Here's how the part is built. I have some questions about the finished solid (model axes, mm). A direction names the side the tool comes from. Give positions to 0.01 mm unless a question says otherwise; leave off trailing zeros. Loops run counter-clockwise (first coordinate to the right, second up) from the corner with the lowest first, then second, coordinate; pieces in that order, holes last. Notation, with made-up numbers: (-37.75, 74) - (-29.75, 74) arc R8 cw to (-29.75, 86) - close; hole circle Ø8 at (86.25, 2). An arc over 180 degrees is marked (long way). Put each result on its own line as item: value. Start each with the question number.
from build123d import *

# Parameters (mm, degrees)
BOSS_EXTRUDE1_DEPTH             = 65
SKETCH2_R                       = 7.5
BOSS_EXTRUDE2_DEPTH             = 2.5
BOSS_EXTRUDE3_REACH             = 88.168
SKETCH3_W                       = 65
SKETCH3_H                       = 3
BOSS_EXTRUDE3_DIRECTION_2_REACH = 88.168
CUT_EXTRUDE2_REACH              = 124.042
SKETCH6_R                       = 1.75
CUT_EXTRUDE3_REACH              = 86.299
CUT_EXTRUDE4_REACH              = 86.299
FILLET1_R                       = 2.5
FILLET2_R                       = 5
CUT_EXTRUDE5_DEPTH              = 111.566721937
CUT_EXTRUDE5_DEPTH_BACK         = 111.566721937
SKETCH9_W                       = 12
SKETCH9_H                       = 32.949220019
SKETCH9_H_2                     = 17.949220019


with BuildPart() as part:
    # Sketch1 → Boss-Extrude1 (new body)
    with BuildSketch(Plane.XY):
        Polygon((-40, 30), (-30, 40), (30, 40), (40, 30), (40, -30), (30, -40), (-30, -40), (-40, -30), align=None)
        Polygon((-37.5, 28.964466094), (-28.964466094, 37.5), (28.964466094, 37.5), (37.5, 28.964466094), (37.5, -28.964466094), (28.964466094, -37.5), (-28.964466094, -37.5), (-37.5, -28.964466094), align=None, mode=Mode.SUBTRACT)
    extrude(amount=BOSS_EXTRUDE1_DEPTH)

    # Sketch2 → Boss-Extrude2 (add)
    with BuildSketch(Plane.XY):
        Polygon((37.5, 28.964466094), (28.964466094, 37.5), (-28.964466094, 37.5), (-37.5, 28.964466094), (-37.5, -28.964466094), (-28.964466094, -37.5), (28.964466094, -37.5), (37.5, -28.964466094), align=None)
        Circle(SKETCH2_R, mode=Mode.SUBTRACT)
    extrude(amount=BOSS_EXTRUDE2_DEPTH)

    # Boss-Extrude3: up to this plane
    boss_extrude3_end = Plane(origin=(28.964466094, 37.5, 65), z_dir=(-0.7071067811865476, -0.7071067811865476, 0))
    # Sketch3 → Boss-Extrude3 (add, up to the surface)
    with BuildSketch(Plane(origin=(0, 0, 0), x_dir=(0, 0, -1), z_dir=(1, 0, 0)), mode=Mode.PRIVATE) as boss_extrude3_sk1:
        with Locations((-32.5, 31)):
            Rectangle(SKETCH3_W, SKETCH3_H)
    boss_extrude3_tool1 = split(extrude(boss_extrude3_sk1.sketch, amount=BOSS_EXTRUDE3_REACH, mode=Mode.PRIVATE), bisect_by=boss_extrude3_end, keep=Keep.BOTH, mode=Mode.PRIVATE)
    add(boss_extrude3_tool1.solids().sort_by_distance((0, 31, 32.5))[0])

    # Boss-Extrude3 direction 2: up to this plane
    boss_extrude3_direction_2_end = Plane(origin=(-37.5, 28.964466094, 65), z_dir=(0.707106781186547, -0.7071067811865481, 0))
    # Sketch3 → Boss-Extrude3 direction 2 (add, up to the surface)
    with BuildSketch(Plane(origin=(0, 0, 0), x_dir=(0, 0, -1), z_dir=(1, 0, 0)), mode=Mode.PRIVATE) as boss_extrude3_direction_2_sk1:
        with Locations((-32.5, 31)):
            Rectangle(SKETCH3_W, SKETCH3_H)
    boss_extrude3_direction_2_tool1 = split(extrude(boss_extrude3_direction_2_sk1.sketch, amount=-BOSS_EXTRUDE3_DIRECTION_2_REACH, mode=Mode.PRIVATE), bisect_by=boss_extrude3_direction_2_end, keep=Keep.BOTH, mode=Mode.PRIVATE)
    add(boss_extrude3_direction_2_tool1.solids().sort_by_distance((0, 31, 32.5))[0])

    # Sketch6 → Cut-Extrude2 (cut, up to next)
    with BuildSketch(Plane(origin=(0, 29.5, -27), x_dir=(-1, 0, 0), z_dir=(0, -1, 0)), mode=Mode.PRIVATE) as cut_extrude2_sk1:
        with Locations(Location((0, -72, 0), (0, 0, 90))):
            Circle(SKETCH6_R)
    cut_extrude2_tool1 = extrude(cut_extrude2_sk1.sketch, amount=-CUT_EXTRUDE2_REACH, mode=Mode.PRIVATE) & part.part
    # Sketch6 → Cut-Extrude2 (cut, up to next)
    with BuildSketch(Plane(origin=(0, 29.5, -27), x_dir=(-1, 0, 0), z_dir=(0, -1, 0)), mode=Mode.PRIVATE) as cut_extrude2_sk2:
        with Locations(Location((30, -37, 0), (0, 0, 90))):
            Circle(SKETCH6_R)
    cut_extrude2_tool2 = extrude(cut_extrude2_sk2.sketch, amount=-CUT_EXTRUDE2_REACH, mode=Mode.PRIVATE) & part.part
    add(cut_extrude2_tool1.solids().sort_by_distance((0, 29.5, 45))[0], mode=Mode.SUBTRACT)
    add(cut_extrude2_tool2.solids().sort_by_distance((-30, 29.5, 10))[0], mode=Mode.SUBTRACT)

    # Sketch7 → Cut-Extrude3 (cut, up to next)
    with BuildSketch(Plane.XY.offset(2.5), mode=Mode.PRIVATE) as cut_extrude3_sk1:
        Polygon((-33.964466094, 32.5), (-28.964466094, 37.5), (28.964466094, 37.5), (33.964466094, 32.5), align=None)
    cut_extrude3_tool1 = extrude(cut_extrude3_sk1.sketch, amount=-CUT_EXTRUDE3_REACH, mode=Mode.PRIVATE) & part.part
    add(cut_extrude3_tool1.solids().sort_by_distance((0, 34.933788, 2.5))[0], mode=Mode.SUBTRACT)

    # Sketch8 → Cut-Extrude4 (cut, up to next)
    with BuildSketch(Plane.XY.offset(2.5), mode=Mode.PRIVATE) as cut_extrude4_sk1:
        with BuildLine():
            Line((-5, 7.5), (0, 7.5))
            Line((0, 7.5), (-7.5, 0))
            ThreePointArc((-7.5, 0), (-8.440285268, 7.256939094), (-15, 10.5))
            Line((-15, 10.5), (-25, 10.5))
            Line((-25, 10.5), (-25, 19.5))
            Line((-25, 19.5), (-5, 19.5))
            Line((-5, 19.5), (-5, 7.5))
        make_face()
    cut_extrude4_tool1 = extrude(cut_extrude4_sk1.sketch, amount=-CUT_EXTRUDE4_REACH, mode=Mode.PRIVATE) & part.part
    add(cut_extrude4_tool1.solids().sort_by_distance((-13.255262, 13.384188, 2.5))[0], mode=Mode.SUBTRACT)

    # Fillet1
    fillet1_edges = [part.edges().sort_by_distance(p)[0] for p in [
        (-25, 10.5, 1.25),
        (-25, 19.5, 1.25),
        (-5, 19.5, 1.25),
    ]]
    fillet(fillet1_edges, radius=FILLET1_R)

    # Fillet2
    fillet2_edges = [part.edges().sort_by_distance(p)[0] for p in [
        (-5, 7.5, 1.25),
    ]]
    fillet(fillet2_edges, radius=FILLET2_R - 0.0001)  # a hair under: the kernel refuses the full size

    # Sketch9 → Cut-Extrude5 (cut, two sides: drawn at the far end of the back side and taken through both)
    with BuildSketch(Plane(origin=(0, 40, 0), x_dir=(1, 0, 0), z_dir=(0, 1, 0)).offset(-CUT_EXTRUDE5_DEPTH_BACK)):
        with Locations((31.5, -66.474610009)):
            Rectangle(SKETCH9_W, SKETCH9_H)
        with Locations((-20, -58.97461001)):
            Rectangle(SKETCH9_W, SKETCH9_H_2)
    extrude(amount=CUT_EXTRUDE5_DEPTH + CUT_EXTRUDE5_DEPTH_BACK, mode=Mode.SUBTRACT)


solid = part.part
1) I'm going to push flat-ended pins straight in: P1, Ø12, axis at x = 20, y = 5, coming from the +Z side; P2, Ø2, axis at y = 38.5, z = 60.5, coming from the +X side; P3, Ø2.5, axis at x = -18.5, y = 31.5, coming from the +Z side. Where does each tip first touch, or does it pass through?
2) Suppose I cut it at A-A on z = 19.5. Please give me the cut outline in (x, y).
3) Suppose I cut it at B-B on x = 14.5. Please give me the cut outline in (y, z).
4) Suppose I cut it at D-D on z = 45. Please give me the cut outline in (x, y), plus the area to 3 significant figures.
5) Thinking about a two-plate mould opening in Y: for faces 4 (the flat face through (-20, 31, 50)), 5 (the flat face through (35, -35, 25)), 6 (the cylindrical face through (-3.5, 8.93, 1.23)), which applies, pulls with the +Y half, pulls with the -Y half, needs draft (parallel to the pull), parting line crosses it, or undercut?
6) Which directions (+Z, -Z, +X, -X, +Y, -Y) give clear straight access to the entire face, cutting with the end or side of a thin tool? Please do faces 1 (the flat face through (33.292, -33.172, 25.917)), 2 (the flat face through (25.5, 31, 58)), 3 (the flat face through (-5, 15, 1)).
7) Suppose I cut it at C-C on y = 0. Please give me the cut outline in (x, z).
8) I need wall thicknesses on line 1 (Y direction, x = 16, z = 32.5); line 2 (Y direction, x = 0, z = 0.55); line 3 (X direction, y = 14.5, z = 49). Which ranges of each line are inside material? Lowest first, please.
Ans:
1. P1: stops at z = 2.5
1. P2: stops at x = 25.5
1. P3: stops at z = 50
2. outline: (-40, -30) - (-30, -40) - (30, -40) - (40, -30) - (40, 30) - (30, 40) - (-30, 40) - (-40, 30) - close; hole (-37.5, -28.96) - (-28.96, -37.5) - (28.96, -37.5) - (37.5, -28.96) - (37.5, 28.96) - (36.96, 29.5) - (-36.96, 29.5) - (-37.5, 28.96) - close; hole (-33.96, 32.5) - (33.96, 32.5) - (28.96, 37.5) - (-28.96, 37.5) - close
3. outline: (-40, 0) - (32.5, 0) - (32.5, 65) - (29.5, 65) - (29.5, 2.5) - (-37.5, 2.5) - (-37.5, 65) - (-40, 65) - close; (37.5, 0) - (40, 0) - (40, 65) - (37.5, 65) - close
4. outline: (-40, -30) - (-30, -40) - (30, -40) - (40, -30) - (40, 30) - (30, 40) - (-30, 40) - (-40, 30) - close; hole (-37.5, -28.96) - (-28.96, -37.5) - (28.96, -37.5) - (37.5, -28.96) - (37.5, 28.96) - (36.96, 29.5) - (1.75, 29.5) - (1.75, 32.5) - (33.96, 32.5) - (28.96, 37.5) - (-28.96, 37.5) - (-33.96, 32.5) - (-1.75, 32.5) - (-1.75, 29.5) - (-36.96, 29.5) - (-37.5, 28.96) - close
4. area: 923 mm²
5. face 4: needs draft
5. face 5: pulls with the -Y half
5. face 6: undercut
6. face 1: +Z
6. face 2: +Z, +Y, -Y
6. face 3: +Z, -Z
7. outline: (-40, 0) - (-7.5, 0) - (-7.5, 2.5) - (-37.5, 2.5) - (-37.5, 65) - (-40, 65) - close; (7.5, 0) - (40, 0) - (40, 65) - (37.5, 65) - (37.5, 2.5) - (7.5, 2.5) - close
8. line 1: y = -40 to -37.5, 29.5 to 32.5, 37.5 to 40
8. line 2: y = -40 to -7.5, 7.5 to 32.5, 37.5 to 40
8. line 3: x = -40 to -37.5, 37.5 to 40
